from build123d import *

# Parameters (mm, degrees)
BOSS_EXTRUDE1_DEPTH     = 24
SKETCH3_R               = 10
BOSS_EXTRUDE2_DEPTH     = 30
CUT_EXTRUDE1_DEPTH      = 77.655071587
CUT_EXTRUDE1_DEPTH_BACK = 77.655071587
SKETCH4_R               = 10
CUT_EXTRUDE2_DEPTH      = 105.76640683
CUT_EXTRUDE2_DEPTH_BACK = 24
SKETCH7_R               = 6
FILLET3_R               = 6


with BuildPart() as part:
    # Sketch2 → Boss-Extrude1 (new body)
    with BuildSketch(Plane(origin=(0, 0, 0), x_dir=(1, 0, 0), z_dir=(0, 1, 0))):
        with BuildLine():
            Line((-24, 12), (40, 12))
            Line((40, 12), (40, -12))
            Line((40, -12), (-24, -12))
            ThreePointArc((-24, -12), (-60, 0), (-24, 12))
        make_face()
    extrude(amount=BOSS_EXTRUDE1_DEPTH)

    # Sketch3 → Boss-Extrude2 (add)
    with BuildSketch(Plane(origin=(40, 0, 0), x_dir=(0, 0, -1), z_dir=(1, 0, 0))):
        with Locations((0, 12)):
            Circle(SKETCH3_R)
    extrude(amount=BOSS_EXTRUDE2_DEPTH)

    # Sketch4 → Cut-Extrude1 (cut, two sides: drawn at the far end of the back side and taken through both)
    with BuildSketch(Plane(origin=(0, 24, 0), x_dir=(1, 0, 0), z_dir=(0, 1, 0)).offset(-CUT_EXTRUDE1_DEPTH_BACK)):
        with Locations(Location((-40, 0, 0), (0, 0, 270))):
            Circle(SKETCH4_R)
    extrude(amount=CUT_EXTRUDE1_DEPTH + CUT_EXTRUDE1_DEPTH_BACK, mode=Mode.SUBTRACT)

    # Sketch7 → Cut-Extrude2 (cut, two sides: drawn at the far end of the back side and taken through both)
    with BuildSketch(Plane(origin=(40, 0, 0), x_dir=(0, 0, -1), z_dir=(1, 0, 0)).offset(-CUT_EXTRUDE2_DEPTH_BACK)):
        with Locations((-12, 24)):
            Circle(SKETCH7_R)
        with Locations((12, 24)):
            Circle(SKETCH7_R)
        with Locations((12, 0)):
            Circle(SKETCH7_R)
        with Locations((-12, 0)):
            Circle(SKETCH7_R)
    extrude(amount=CUT_EXTRUDE2_DEPTH + CUT_EXTRUDE2_DEPTH_BACK, mode=Mode.SUBTRACT)

    # Fillet3
    fillet3_edges = [part.edges().sort_by_distance(p)[0] for p in [
        (16, 4.242640687, -7.757359313),
        (16, 4.242640687, 7.757359313),
        (16, 19.757359313, -7.757359313),
        (16, 19.757359313, 7.757359313),
    ]]
    fillet(fillet3_edges, radius=FILLET3_R - 0.0001)  # a hair under: the kernel refuses the full size


solid = part.part
Verification items for the finished model (mm, model axes). A direction names the side the tool comes from. Round coordinates to 2 decimals unless told otherwise and drop trailing zeros. Order: outer loops, then holes, each group sorted by start corner. A loop starts at its lowest first (then second) coordinate and runs counter-clockwise, first axis right, second up.
1. Section check B-B on z = 0. Record the cut outline in (x, y), then the cut area to 3 significant figures.
Final values:
outline: (-60, 0) - (-50, 0) - (-50, 24) - (-60, 24) - close; (-30, 0) - (40, 0) - (40, 2) - (70, 2) - (70, 22) - (40, 22) - (40, 24) - (-30, 24) - close
area: 2,520 mm2
2. Section check D-D on x = -6.5. Record the cut outline in (y, z).
Final values:
outline: (0, -12) - (24, -12) - (24, 12) - (0, 12) - close
3. Thickness scan on L1, parallel to X at y = 13.25, z = 0; L2, parallel to Z at x = -40, y = 17; L3, parallel to Z at x = 24, y = 7. Record the ranges inside material, lowest first.
Final values:
L1: x = -60 to -50, -30 to 70
L2: z = -20 to -10, 10 to 20
L3: z = -12 to 12
4. Section check A-A on x = -40. Record the cut outline in (y, z), then the cut area to 3 significant figures.
Final values:
outline: (0, -20) - (24, -20) - (24, -10) - (0, -10) - close; (0, 10) - (24, 10) - (24, 20) - (0, 20) - close
area: 480 mm2
5. Access from +Z, -Z, +X, -X, +Y, -Y to the whole of each face (thin tool, end or side, straight path). Record for faces 1 (the flat face through (0, 12, -12)), 2 (the cylindrical face through (54.79, 2.24, 2.17)), 3 (the cylindrical face through (30.874, 4.196, 7.711)), 4 (the cylindrical face through (30.874, 4.289, -7.804)).
Final values:
face 1: -Z, +X, +Y, -Y
face 2: +X
face 3: +Z, +X, -Y
face 4: -Z, +X, -Y
6. Go/stop test with flat-tipped pins: P1, Ø10, axis at y = 5.5, z = -14.5, coming from the -X side; P2, Ø8, axis at x = 20, y = 6.5, coming from the +Z side; P3, Ø12, axis at x = 12.5, y = 8.5, coming from the -Z side; P4, Ø1, axis at x = 41, z = -13.5, coming from the -Y side. Record where each tip stops, or that it passes through.
Final values:
P1: stops at x = -57.6
P2: stops at z = 12
P3: stops at z = -12
P4: passes through
7. Release check for a two-part mould opening along Z. For faces 5 (the flat face through (1, 12, 12)), 6 (the flat face through (-9, 24, 0)), 7 (the cylindrical face through (30.874, 19.804, -7.711)), 8 (the cylindrical face through (-49.76, 11.83, -2.17)) record: +Z half, -Z half, draft (parallel to the pull), parting line (faces both ways), or undercut.
Final values:
face 5: +Z half
face 6: draft
face 7: -Z half
face 8: undercut
8. Section check C-C on y = 12. Record the cut outline in (x, z), then the cut area to 3 significant figures.
Final values:
outline: (-24, -12) - (40, -12) - (40, -10) - (70, -10) - (70, 10) - (40, 10) - (40, 12) - (-24, 12) arc R20 ccw (long way) to start; hole circle Ø20 at (-40, 0)
area: 3,010 mm2
